```python
from build123d import *

# Parameters (mm, degrees)
SKETCH_R  = 5.5
PAD_DEPTH = 6


with BuildPart() as part:
    # Sketch → Pad (new body)
    with BuildSketch(Plane.YZ):
        Polygon((-26, 35.5), (26, 35.5), (35, 26.5), (35, 5.5), (-35, 5.5), (-35, 26.5), align=None)
        with Locations((-20, 20.5)):
            Circle(SKETCH_R, mode=Mode.SUBTRACT)
        with Locations((20, 20.5)):
            Circle(SKETCH_R, mode=Mode.SUBTRACT)
    extrude(amount=PAD_DEPTH)


solid = part.part
```
The listing builds one solid part. Answer for the finished solid, in the listing's coordinates (mm). Round coordinates to 2 decimals unless told otherwise and drop trailing zeros. Loops run counter-clockwise (first coordinate to the right, second up) from the corner with the lowest first, then second, coordinate; pieces in that order, holes last.
Q1. For a pull along Z with two mould halves and no side action, classify faces 1 (the face through (3, 0, 35.5)), 2 (the face through (3, 0, 5.5)), 3 (the face through (2.958, -14.754, 22.152)) as released by +Z, released by -Z, zero draft, split by the parting line, or undercut.
Q2. Section A-A, the plane z = 20.5 is taken. Determine the outline of the cut face in (x, y), then the cut area to 3 significant figures.
Q3. Section B-B, the plane y = 20 is taken. Determine the outline of the cut face in (x, z).
Q4. Find the intervals of material crossed by line 1 (Z direction, x = 4.6, y = -20); line 2 (Y direction, x = 1.1, z = 22.5); line 3 (Y direction, x = 4.95, z = 22.75), in increasing order.
Q5. Section C-C, the plane x = 2.95 is taken. Determine the outline of the cut face in (y, z), then the cut area to 3 significant figures.
Q6. Section D-D, the plane y = -17.5 is taken. Determine the outline of the cut face in (x, z).
Q7. Given pin 1 Ø9 at (y, z) = (-20, 20.5) entering from -X, flat-ended and moving along its own axis, determine where the tip first touches the part or whether it passes through.
Completed:
1. face 1: released by +Z
1. face 2: released by -Z
1. face 3: undercut
2. outline: (0, -35) - (6, -35) - (6, -25.5) - (0, -25.5) - close; (0, -14.5) - (6, -14.5) - (6, 14.5) - (0, 14.5) - close; (0, 25.5) - (6, 25.5) - (6, 35) - (0, 35) - close
2. area: 288 mm2
3. outline: (0, 5.5) - (6, 5.5) - (6, 15) - (0, 15) - close; (0, 26) - (6, 26) - (6, 35.5) - (0, 35.5) - close
4. line 1: z = 5.5 to 15, 26 to 35.5
4. line 2: y = -35 to -25.12, -14.88 to 14.88, 25.12 to 35
4. line 3: y = -35 to -25.02, -14.98 to 14.98, 25.02 to 35
5. outline: (-35, 5.5) - (35, 5.5) - (35, 26.5) - (26, 35.5) - (-26, 35.5) - (-35, 26.5) - close; hole circle Ø11 at (-20, 20.5); hole circle Ø11 at (20, 20.5)
5. area: 1,830 mm2
6. outline: (0, 5.5) - (6, 5.5) - (6, 15.6) - (0, 15.6) - close; (0, 25.4) - (6, 25.4) - (6, 35.5) - (0, 35.5) - close
7. pin 1: passes through
